Source: CAD feature listing. Evaluate the final solid. Frame: model axes, mm. A direction names the side the tool comes from. Round coordinates to 2 decimals unless told otherwise and drop trailing zeros. Answer in a Markdown table with one row per item.
from build123d import *

# Parameters (mm, degrees)
SKETCH1_W           = 152.4
SKETCH1_H           = 127
BOSS_EXTRUDE1_DEPTH = 3.048
SKETCH2_W           = 6.35
SKETCH2_H           = 3.048
CUT_EXTRUDE1_DEPTH  = 100.236990603


with BuildPart() as part:
    # Sketch1 → Boss-Extrude1 (new body)
    with BuildSketch(Plane(origin=(0, 0, 0), x_dir=(1, 0, 0), z_dir=(0, 1, 0))):
        Rectangle(SKETCH1_W, SKETCH1_H)
    extrude(amount=BOSS_EXTRUDE1_DEPTH)

    # Sketch2 → Cut-Extrude1 (cut, through all)
    with BuildSketch(Plane(origin=(0, 3.048, 0), x_dir=(1, 0, 0), z_dir=(0, 1, 0))):
        with Locations((-66.675, -61.976)):
            Rectangle(SKETCH2_W, SKETCH2_H)
        with Locations((-53.975, -61.976)):
            Rectangle(SKETCH2_W, SKETCH2_H)
        with Locations((-41.275, -61.976)):
            Rectangle(SKETCH2_W, SKETCH2_H)
        with Locations((-28.575, -61.976)):
            Rectangle(SKETCH2_W, SKETCH2_H)
        with Locations((-15.875, -61.976)):
            Rectangle(SKETCH2_W, SKETCH2_H)
        with Locations((-3.175, -61.976)):
            Rectangle(SKETCH2_W, SKETCH2_H)
        with Locations((9.525, -61.976)):
            Rectangle(SKETCH2_W, SKETCH2_H)
        with Locations((22.225, -61.976)):
            Rectangle(SKETCH2_W, SKETCH2_H)
        with Locations((47.625, -61.976)):
            Rectangle(SKETCH2_W, SKETCH2_H)
        with Locations((60.325, -61.976)):
            Rectangle(SKETCH2_W, SKETCH2_H)
        with Locations((34.925, -61.976)):
            Rectangle(SKETCH2_W, SKETCH2_H)
        with Locations((73.025, -61.976)):
            Rectangle(SKETCH2_W, SKETCH2_H)
        with Locations((-66.675, 61.976)):
            Rectangle(SKETCH2_W, SKETCH2_H)
        with Locations((-53.975, 61.976)):
            Rectangle(SKETCH2_W, SKETCH2_H)
        with Locations((-41.275, 61.976)):
            Rectangle(SKETCH2_W, SKETCH2_H)
        with Locations((-28.575, 61.976)):
            Rectangle(SKETCH2_W, SKETCH2_H)
        with Locations((-15.875, 61.976)):
            Rectangle(SKETCH2_W, SKETCH2_H)
        with Locations((-3.175, 61.976)):
            Rectangle(SKETCH2_W, SKETCH2_H)
        with Locations((9.525, 61.976)):
            Rectangle(SKETCH2_W, SKETCH2_H)
        with Locations((22.225, 61.976)):
            Rectangle(SKETCH2_W, SKETCH2_H)
        with Locations((34.925, 61.976)):
            Rectangle(SKETCH2_W, SKETCH2_H)
        with Locations((47.625, 61.976)):
            Rectangle(SKETCH2_W, SKETCH2_H)
        with Locations((60.325, 61.976)):
            Rectangle(SKETCH2_W, SKETCH2_H)
        with Locations((73.025, 61.976)):
            Rectangle(SKETCH2_W, SKETCH2_H)
    extrude(amount=-CUT_EXTRUDE1_DEPTH, mode=Mode.SUBTRACT)


solid = part.part
Q1. Pull-direction query (X, two-part tool) for faces 1 (the flat face through (38.1, 2, -62)), 2 (the flat face through (73, 2, 60.452)); classes: pulls with the +X half, pulls with the -X half, needs draft (parallel to the pull), parting line crosses it, or undercut.
Solutions:
| item | result |
|---|---|
| face 1 | undercut |
| face 2 | needs draft |
Q2. Material intervals for probe 1 along Z at (x, y) = (-38.5, 1.6), sorted ascending.
Solutions:
| item | result |
|---|---|
| probe 1 | z = -60.45 to 60.45 |
Q3. Contact query for flat-ended pins moving along their axis: pin 1 Ø1.5 at (x, y) = (-55.5, 2) entering from -Z; pin 2 Ø1.5 at (y, z) = (2, 62) entering from +X. Output: stop coordinate, or through.
Solutions:
| item | result |
|---|---|
| pin 1 | stops at z = -60.45 |
| pin 2 | stops at x = 69.85 |
Q4. Access query for faces 3 (the flat face through (-6.35, 2, 62)), 4 (the flat face through (54, 2, -63.5)), 5 (the flat face through (-54, 2, -60.452)). Directions: +Z, -Z, +X, -X, +Y, -Y. A direction counts if a zero-diameter tool reaches every point of the face in a straight line with its end or side. Return the directions, or none.
Solutions:
| item | result |
|---|---|
| face 3 | +Z, +Y, -Y |
| face 4 | -Z, +X, -X, +Y, -Y |
| face 5 | -Z, +Y, -Y |
